For this review, take the finished solid that the model builds, in its own axes (mm). A direction names the side the tool comes from. Coordinates: 2 decimals unless noted, no trailing zeros. Loops run counter-clockwise (first coordinate to the right, second up) from the corner with the lowest first, then second, coordinate; pieces in that order, holes last. Notation, with made-up numbers: M -18.75,-14 L 30.25,-14 A19 ccw 30.25,13 Z; hole C 80,73 d9. An arc over 180 degrees is marked long. Write item = value, one per line.
from build123d import *

# Parameters (mm, degrees)
F0_R      = 49
F0_R_2    = 6
F1_DEPTH  = 15
F2_R      = 25.016122
F3_DEPTH  = 75
F4_R      = 6
F5_DEPTH  = 15
F6_R      = 17.5
F7_DEPTH  = 30
F9_R      = 13
F10_DEPTH = 150


with BuildPart() as f1:
    # F0 (on Top) → F1 (new body)
    with BuildSketch(Plane.XY):
        Circle(F0_R)
        with Locations((0, -35)):
            Circle(F0_R_2, mode=Mode.SUBTRACT)
        with Locations((-30.310889, -17.5)):
            Circle(F0_R_2, mode=Mode.SUBTRACT)
        with Locations((30.310889, -17.5)):
            Circle(F0_R_2, mode=Mode.SUBTRACT)
        with Locations((-30.310889, 17.5)):
            Circle(F0_R_2, mode=Mode.SUBTRACT)
        with Locations((0, 35)):
            Circle(F0_R_2, mode=Mode.SUBTRACT)
        with Locations((30.310889, 17.5)):
            Circle(F0_R_2, mode=Mode.SUBTRACT)
    extrude(amount=F1_DEPTH)

    # F2 (on face) → F3 (join)
    with BuildSketch(Plane.XY.offset(15)):
        Circle(F2_R)
    extrude(amount=F3_DEPTH)

    # F4 (on face) → F5 (join)
    with BuildSketch(Plane.XY.offset(90)):
        with BuildLine():
            Line((9, -28.618176), (54.5, -14.309088))
            ThreePointArc((54.5, -14.309088), (65, 0), (54.5, 14.309088))
            Line((54.5, 14.309088), (9, 28.618176))
            ThreePointArc((9, 28.618176), (0, 30), (-9, 28.618176))
            Line((-9, 28.618176), (-54.5, 14.309088))
            ThreePointArc((-54.5, 14.309088), (-65, 0), (-54.5, -14.309088))
            Line((-54.5, -14.309088), (-9, -28.618176))
            ThreePointArc((-9, -28.618176), (0, -30), (9, -28.618176))
        make_face()
        with Locations((-50, 0)):
            Circle(F4_R, mode=Mode.SUBTRACT)
        with Locations((50, 0)):
            Circle(F4_R, mode=Mode.SUBTRACT)
    extrude(amount=F5_DEPTH)


with BuildPart() as f7:
    # F6 (on face) → F7 (new body)
    with BuildSketch(Plane.XY.offset(105)):
        Circle(F6_R)
    extrude(amount=-F7_DEPTH)


with BuildPart() as f1_1:
    add(f1.part)

    # F8: cut F7
    add(f7.part, mode=Mode.SUBTRACT)


with BuildPart() as f10:
    # F9 (on face) → F10 (new body)
    with BuildSketch(Plane.XY.offset(75)):
        Circle(F9_R)
    extrude(amount=-F10_DEPTH)


with BuildPart() as f1_2:
    add(f1_1.part)

    # F11: cut F10
    add(f10.part, mode=Mode.SUBTRACT)


solid = f1_2.part
Q1. Draft analysis for pull direction Z (two halves, no side actions). For faces 1 (the face through (-31.432, 21.564, 97.395)), 2 (the face through (14, -13, 105)), 3 (the face through (-24.99, 1.1, 51.98)), state which applies: +Z half, -Z half, draft (parallel to the pull), parting line (faces both ways), or undercut.
Solved:
face_1 = draft
face_2 = +Z half
face_3 = undercut
Q2. For line 1 along Y through (x, z) = (-6, 37); line 2 along Y through (x, z) = (0, 90.5); line 3 along Z through (x, y) = (35.5, -23), list the stretches that pass through material, from the lowest coordinate up.
Solved:
line_1 = -24.29 to -11.53, 11.53 to 24.29
line_2 = -30 to -17.5, 17.5 to 30
line_3 = 0 to 15
Q3. Add section A-A (x = 27). Write out the cut boundary in (y, z), and give its area (3 significant figures).
Solved:
outline = M -40.89,0 L -22.5,0 L -22.5,15 L -40.89,15 Z; M -22.96,90 L 22.96,90 L 22.96,105 L -22.96,105 Z; M -12.5,0 L 12.5,0 L 12.5,15 L -12.5,15 Z; M 22.5,0 L 40.89,0 L 40.89,15 L 22.5,15 Z
area = 1,620 mm²
Q4. Add section C-C (y = 35). Write out the cut boundary in (x, z).
Solved:
outline = M -34.29,0 L -6,0 L -6,15 L -34.29,15 Z; M 6,0 L 34.29,0 L 34.29,15 L 6,15 Z
Q5. For pin 1 Ø11 at (x, y) = (50, 0) entering from +Z; pin 2 Ø5 at (x, z) = (-16, 88) entering from -Y; pin 3 Ø9.5 at (x, y) = (-30.31, -17.5) entering from -Z, all flat-tipped, find the tip position at first contact; note any pin that passes through.
Solved:
pin_1 = 15
pin_2 = -26.89
pin_3 = 90
Q6. Add section B-B (y = 3). Write out the cut boundary in (x, z), and give its area (3 significant figures).
Solved:
outline = M -64.7,90 L -55.2,90 L -55.2,105 L -64.7,105 Z; M -48.91,0 L -12.65,0 L -12.65,75 L -17.24,75 L -17.24,105 L -44.8,105 L -44.8,90 L -24.84,90 L -24.84,15 L -48.91,15 Z; M 12.65,0 L 48.91,0 L 48.91,15 L 24.84,15 L 24.84,90 L 44.8,90 L 44.8,105 L 17.24,105 L 17.24,75 L 12.65,75 Z; M 55.2,90 L 64.7,90 L 64.7,105 L 55.2,105 Z
area = 3,890 mm²
Q7. Machinability: for faces 4 (the face through (-1.301, 29.143, 7.395)), 5 (the face through (-56, 0, 97)), 6 (the face through (32.068, 21.363, 97.395)), 7 (the face through (0, 30, 97)), which of the approach directions +Z, -Z, +X, -X, +Y, -Y give a long, thin tool a straight path to every point of the face, cutting with its end or side? Answer none if there is none.
Solved:
face_4 = -Z
face_5 = +Z
face_6 = +Z, +X, +Y
face_7 = +Z, +Y
Q8. Add section D-D (z = 56.5). Write out the cut boundary in (x, y), and give its area (3 significant figures).
Solved:
outline = C 0,0 d50.03; hole C 0,0 d26
area = 1,440 mm²
